Geometry check sheet. Reference: the model listing, model coordinates, mm. A direction names the side the tool comes from. Coordinates: 2 decimals unless noted, no trailing zeros. Write each loop counter-clockwise with the first axis right and the second up, starting at its lowest first coordinate (ties: lowest second). Pieces come first, ordered by that corner, then holes. Notation, with made-up numbers: (-27.5, -24.5) -> (-13.5, -24.5) arc R13 ccw to (-13.5, 0.5) -> close; hole circle Ø1 at (-9, 35.25). An arc over 180 degrees is marked (long way). One line per question, with ' | ' between items.
```python
from build123d import *

# Parameters (mm, degrees)
F1_DEPTH      = 28.575
F2_W          = 12.7
F2_H          = 38.1
F3_DEPTH      = 25.4
F3_DEPTH_BACK = 25.4
F4_R          = 1.19126
F5_DEPTH      = 25.4
F5_DEPTH_BACK = 25.4
F6_W          = 6.35
F6_H          = 25.4
F7_DEPTH      = 0.8128
F8_R          = 1.016
F9_DEPTH      = 25.4
F9_DEPTH_BACK = 25.4


with BuildPart() as f1:
    # F0 (on Front) → F1 (new body)
    with BuildSketch(Plane.XZ):
        Polygon((0, 11.1125), (0, 0), (12.7, 0), (12.7, 11.1125), (9.525, 11.1125), (9.525, 3.175), (3.175, 3.175), (3.175, 11.1125), align=None)
    extrude(amount=-F1_DEPTH)

    # F2 (on Top) → F3 (cut, two sides)
    with BuildSketch(Plane.XY) as f3_sk:
        with Locations((15.748, 1.5875)):
            Rectangle(F2_W, F2_H)
    extrude(amount=F3_DEPTH, mode=Mode.SUBTRACT)
    extrude(f3_sk.sketch, amount=-F3_DEPTH_BACK, mode=Mode.SUBTRACT)

    # F4 (on Right) → F5 (cut, two sides)
    with BuildSketch(Plane.YZ) as f5_sk:
        with Locations((8.73252, 5.36321)):
            Circle(F4_R)
        with Locations((24.60752, 5.36321)):
            Circle(F4_R)
        with BuildLine():
            ThreePointArc((2.38252, 4.62661), (1.9155466817, 3.4992366817), (3.04292, 3.96621))
            ThreePointArc((3.04292, 3.96621), (2.8494933183, 4.4331833183), (2.38252, 4.62661))
        make_face()
        with BuildLine():
            ThreePointArc((3.04292, 6.76021), (1.9155466817, 7.2271833183), (2.38252, 6.09981))
            ThreePointArc((2.38252, 6.09981), (2.8494933183, 6.2932366817), (3.04292, 6.76021))
        make_face()
    extrude(amount=F5_DEPTH, mode=Mode.SUBTRACT)
    extrude(f5_sk.sketch, amount=-F5_DEPTH_BACK, mode=Mode.SUBTRACT)

    # F6 (on Right) → F7 (cut)
    with BuildSketch(Plane.YZ):
        with Locations((8.73252, 10.0369287327)):
            Rectangle(F6_W, F6_H)
    extrude(amount=F7_DEPTH, mode=Mode.SUBTRACT)

    # F8 (on Top) → F9 (cut, two sides)
    with BuildSketch(Plane.XY) as f9_sk:
        with Locations((6.35, 20.955)):
            Circle(F8_R)
        with Locations((6.35, 7.62)):
            Circle(F8_R)
    extrude(amount=-F9_DEPTH, mode=Mode.SUBTRACT)
    extrude(f9_sk.sketch, amount=F9_DEPTH_BACK, mode=Mode.SUBTRACT)


solid = f1.part
```
(1) Material ranges on line 1 (X direction, y = 27, z = 10.75) (3 decimals); line 2 (Y direction, x = 10.5, z = 9.25) (1 decimal); line 3 (X direction, y = 12.75, z = 1), recorded low to high.
Answers below:
line 1: x = 0 to 3.175, 9.525 to 12.7 | line 2: y = 20.6 to 28.6 | line 3: x = 0 to 9.4
(2) Depth check by flat-ended pin: P1, Ø1, axis at y = 15, z = 2, coming from the +X side; P2, Ø4, axis at x = 5.5, y = 14.5, coming from the -Z side; P3, Ø2, axis at y = 8.73, z = 5.36, coming from the +X side. Enter the tip coordinate at first touch or a pass-through.
Answers below:
P1: stops at x = 9.4 | P2: stops at z = 0 | P3: passes through
(3) Cross-section at A-A (z = 9). Record the cut outline in (x, y) (1 decimal), plus the area to 3 significant figures.
Answers below:
outline: (0, 0) -> (3.2, 0) -> (3.2, 28.6) -> (0, 28.6) -> (0, 11.9) -> (0.8, 11.9) -> (0.8, 5.6) -> (0, 5.6) -> close; (9.5, 20.6) -> (12.7, 20.6) -> (12.7, 28.6) -> (9.5, 28.6) -> close | area: 111 mm²
(4) Tool access check on faces 1 (the face through (11, 20.638, 5)), 2 (the face through (0.4, 5.558, 5.5)), 3 (the face through (2, 14, 11.112)). Record the directions out of +Z, -Z, +X, -X, +Y, -Y that give a thin tool (end or side, any length) a straight path to the whole face; none if there is none.
Answers below:
face 1: +Z, -Z, +X, -Y | face 2: +Z, -Z, -X | face 3: +Z, +X, -X, +Y, -Y
(5) Cross-section at B-B (x = 6.35). Record the cut outline in (y, z) (3 decimals).
Answers below:
outline: (0, 0) -> (6.604, 0) -> (6.604, 3.175) -> (0, 3.175) -> close; (8.636, 0) -> (19.939, 0) -> (19.939, 3.175) -> (8.636, 3.175) -> close; (21.971, 0) -> (28.575, 0) -> (28.575, 3.175) -> (21.971, 3.175) -> close
(6) Cross-section at C-C (y = 25). Record the cut outline in (x, z) (1 decimal), plus the area to 3 significant figures.
Answers below:
outline: (0, 0) -> (12.7, 0) -> (12.7, 4.2) -> (9.5, 4.2) -> (9.5, 3.2) -> (3.2, 3.2) -> (3.2, 4.2) -> (0, 4.2) -> close; (0, 6.5) -> (3.2, 6.5) -> (3.2, 11.1) -> (0, 11.1) -> close; (9.5, 6.5) -> (12.7, 6.5) -> (12.7, 11.1) -> (9.5, 11.1) -> close | area: 76.4 mm²
(7) Draft check along X on faces 4 (the face through (0, 3, 6)), 5 (the face through (3.175, 14, 7)), 6 (the face through (6, 28.575, 3)), 7 (the face through (6, 14, 3.175)). Enter one of: pulls with the +X half, pulls with the -X half, needs draft (parallel to the pull), parting line crosses it, or undercut.
Answers below:
face 4: pulls with the -X half | face 5: undercut | face 6: needs draft | face 7: undercut
(8) Cross-section at D-D (z = 2). Count the separate pieces of the cut face and the enclosed holes in it, plus the area to 3 significant figures.
Answers below:
separate pieces: 1 | enclosed holes: 2 | area: 283 mm²
